The figure shows three views and two pictorial views of one solid part (mm, origin at its lowest corner). Answer the questions. A direction names the side the tool comes from. Round coordinates to 2 decimals unless told otherwise and drop trailing zeros. Order: outer loops, then holes, each group sorted by start corner. A loop starts at its lowest first (then second) coordinate and runs counter-clockwise, first axis right, second up. Notation, with made-up numbers: M 18.25,55.25 L 48.25,55.25 A26 cw 48.25,71.25 Z; hole C 60,-13 d1. An arc over 180 degrees is marked long. Return JSON: item names as keys, results as strings.
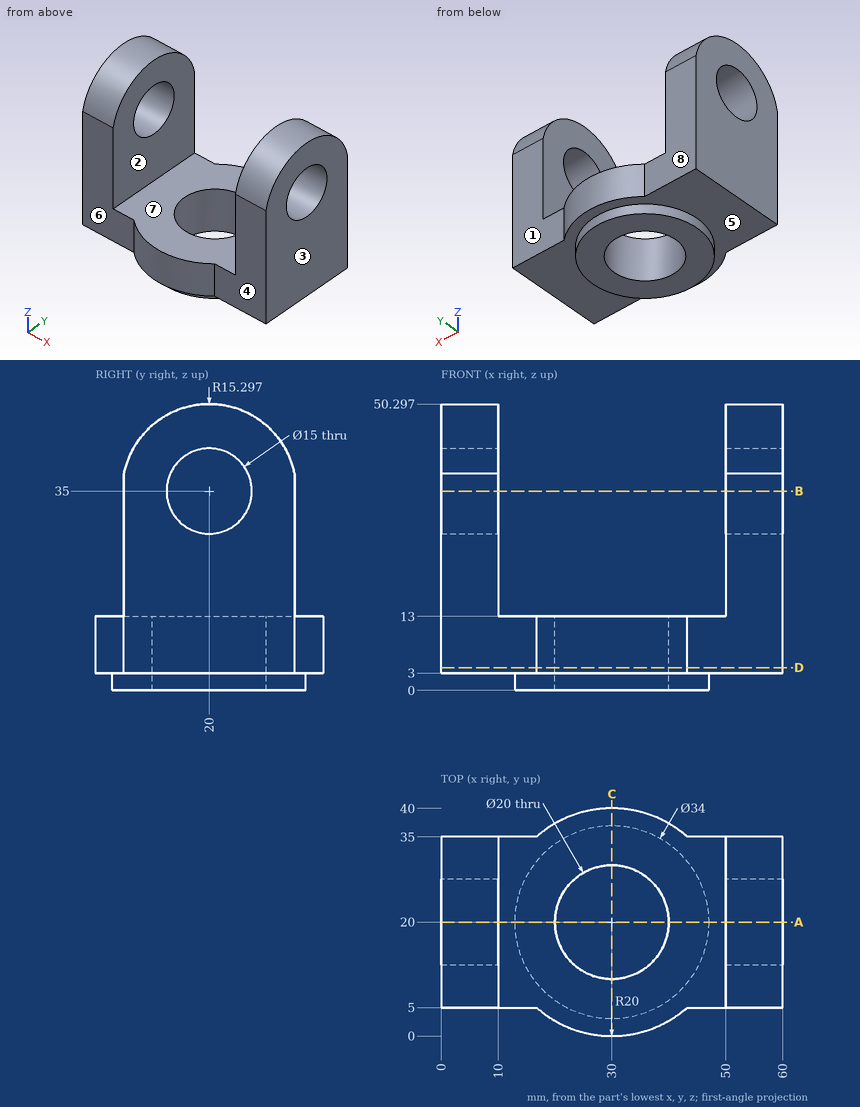
Item 1: Which of the six approach directions +Z, -Z, +X, -X, +Y, -Y give full straight-line access (tool end or side, diameter ignored) to the marked faces 4, 5, 6, 7 and 8?
Output:
{"face 4": "+Z, -Z, +X, -Y", "face 5": "-Z", "face 6": "+Z, -Z, -X, -Y", "face 7": "+Z, +Y, -Y", "face 8": "+Z, -Z, -X, +Y"}
Item 2: Find section C-C (x = 30). Determine the outline of the cut face in (y, z), plus the area to 3 significant figures.
Output:
{"outline": "M 0,3 L 3,3 L 3,0 L 10,0 L 10,13 L 0,13 Z; M 30,0 L 37,0 L 37,3 L 40,3 L 40,13 L 30,13 Z", "area": "242 mm^2"}
Item 3: Find section B-B (z = 35). Determine the outline of the cut face in (x, y).
Output:
{"outline": "M 0,5 L 10,5 L 10,12.5 L 0,12.5 Z; M 0,27.5 L 10,27.5 L 10,35 L 0,35 Z; M 50,5 L 60,5 L 60,12.5 L 50,12.5 Z; M 50,27.5 L 60,27.5 L 60,35 L 50,35 Z"}
Item 4: Consider line 1 along X through (y, z) = (34.5, 26.5); line 2 along X through (y, z) = (20, 7.25); line 3 along Y through (x, z) = (30, 10). Determine where each line is inside the solid, lowest interval first. Write a range as [from, to].
Output:
{"line 1": "x = [0, 10], [50, 60]", "line 2": "x = [0, 20], [40, 60]", "line 3": "y = [0, 10], [30, 40]"}
Item 5: The mould has two halves that part along X. Classify the marked faces 1, 2 and 3: pulls with the +X half, pulls with the -X half, needs draft (parallel to the pull), parting line crosses it, or undercut.
Output:
{"face 1": "needs draft", "face 2": "undercut", "face 3": "pulls with the +X half"}
Item 6: Find section D-D (z = 4). Determine the outline of the cut face in (x, y).
Output:
{"outline": "M 0,5 L 16.77,5 A20 ccw 43.23,5 L 60,5 L 60,35 L 43.23,35 A20 ccw 16.77,35 L 0,35 Z; hole C 30,20 d20"}
Item 7: Find section A-A (y = 20). Determine the outline of the cut face in (x, z).
Output:
{"outline": "M 0,3 L 13,3 L 13,0 L 20,0 L 20,13 L 10,13 L 10,27.5 L 0,27.5 Z; M 0,42.5 L 10,42.5 L 10,50.3 L 0,50.3 Z; M 40,0 L 47,0 L 47,3 L 60,3 L 60,27.5 L 50,27.5 L 50,13 L 40,13 Z; M 50,42.5 L 60,42.5 L 60,50.3 L 50,50.3 Z"}
Item 8: Each of these flat-tipped pins is pushed along its axis until it touches: pin 1 (18 mm diameter, centred on x = 30, y = 20, fed in from +Z); pin 2 (8.5 mm diameter, centred on x = 4.5, z = 18, fed in from +Y); pin 3 (18.5 mm diameter, centred on x = 11, z = 14, fed in from -Y); pin 4 (12 mm diameter, centred on x = 29.5, y = 12, fed in from +Z). Where does it stop, or does it pass through?
Output:
{"pin 1": "passes through", "pin 2": "stops at y = 35", "pin 3": "stops at y = 2.57", "pin 4": "stops at z = 13"}
